Model file for the job. Use its own axes, mm. Round coordinates to 2 decimals unless told otherwise and drop trailing zeros. Order: outer loops, then holes, each group sorted by start corner. A loop starts at its lowest first (then second) coordinate and runs counter-clockwise, first axis right, second up. Notation, with made-up numbers: (-37.75, 45.5) -> (11.25, 45.5) arc R25 cw to (11.25, 82.5) -> close; hole circle Ø9 at (51, -7.75). An arc over 180 degrees is marked (long way). Put each result on its own line as item: value. Start each with the question number.
Q1. Flat gauge pins, fed straight in: P1, Ø0.5, axis at x = -22, y = 0, coming from the +Z side; P2, Ø3, axis at x = -13, z = 2.5, coming from the +Y side; P3, Ø0.7, axis at x = -22.5, y = 1, coming from the -Z side. Where does each tip first touch, or does it go through?
Q2. Cut at A-A, the plane x = -18. List the corners of the cut face in (y, z), and give its area (3 significant figures).
Q3. Pull direction Z, two halves, no side cores. Call faces 1 (the face through (1.5, -0.2, 0.9)), 2 (the face through (-22.575, -0.6, 2.1)), 3 (the face through (-21.975, 0, 1)): released by +Z, released by -Z, zero draft, split by the parting line, or undercut.
Q4. Probe L1, parallel to X at y = 1.8, z = 2.35; L2, parallel to Y at x = -1.75, z = 1.5; L3, parallel to Y at x = -5, z = 0.5. List the from-to ranges inside material, lowest first.
Autodesk Inventor part; units mm, degrees
ref_plane "YZ Plane" through (0, 0, 0) normal (1, 0, 0) x (0, 1, 0)
ref_plane "XZ Plane" through (0, 0, 0) normal (0, 1, 0) x (-1, 0, 0)
ref_plane "XY Plane" through (0, 0, 0) normal (0, 0, 1) x (1, 0, 0)
sketch "Skizze1" plane through (0, 0, 0) normal (0, 1, 0) x (-1, 0, 0)
  line L0 (0, 0) -> (21.1609, 0)
  line L1 (0, 0) -> (-2.4249, 1.4)
  line L2 (0, 0) -> (2.8, 0) construction
  line L3 (21.868, -0.2929) -> (22.5751, -1)
  line L4 (-2.4249, 1.4) -> (-2.4249, 1.5)
  line L5 (-2.4249, 1.5) -> (22.5751, 1.5)
  line L6 (22.5751, -1) -> (22.5751, 1.5)
  arc A0 (21.868, -0.2929) -> (21.1609, 0) centre (21.1609, -1) ccw
  point P0 (21.5751, 0)
  dimension "d22" = 0.1
  dimension "d23" = 25
  dimension "d32" = 1
  dimension "d52" = 1.5
  dimension "d53" = 135
  dimension "d54" = 2.5
  dimension "d55" = 30
revolve "Umdrehung1" add sketch "Skizze1" angle 360 about axis through (2.4249, 0, 1.5) along (-1, 0, 0)
thread "Gewinde1"
sketch "Skizze2" plane through (-22.5751, 0, 1.5) normal (-1, 0, 0) x (0, 0, 1)
  circle A0 centre (0, 0) radius 0.0008
  line L0 (0.4, 1.8) -> (-0.4, 1.8)
  line L1 (0.4, -1.8) -> (-0.4, -1.8)
  line L2 (1.8, 0.4) -> (1.8, -0.4)
  line L3 (-1.8, 0.4) -> (-1.8, -0.4)
  line L4 (-1.8, -0.4) -> (-0.4, -0.4)
  line L5 (-1.8, 0.4) -> (-0.4, 0.4)
  line L6 (1.8, 0.4) -> (0.4, 0.4)
  line L7 (1.8, -0.4) -> (0.4, -0.4)
  line L8 (0.4, -1.8) -> (0.4, -0.4)
  line L9 (0.4, 0.4) -> (0.4, 1.8)
  line L10 (-0.4, -1.8) -> (-0.4, -0.4)
  line L11 (-0.4, 0.4) -> (-0.4, 1.8)
  point P0 (-1.5, 0)
  dimension "d48" = 0.8
  dimension "d49" = 0.8
  dimension "d56" = 1.8
  dimension "d57" = 1.8
  dimension "d58" = 1.8
  dimension "d59" = 1.8
  dimension "d61" = 0.8
  dimension "d62" = 0.8
  dimension "d63" = 0.4
  dimension "d64" = 0.4
  dimension "d65" = 0.4
  dimension "d66" = 0.4
extrude "Extrusion2" cut sketch "Skizze2" against normal blind 0.6
properties part number "Wettterstation_Schraube" material "Edelstahl"
Ans:
1. P1: stops at z = 3.67
1. P2: stops at y = 1.5
1. P3: stops at z = -0.91
2. outline: circle Ø3 at (0, 1.5)
2. area: 7.07 mm^2
3. face 1: split by the parting line
3. face 2: zero draft
3. face 3: undercut
4. L1: x = -22.58 to -22.07
4. L2: y = -1.5 to 1.5
4. L3: y = -1.12 to 1.12
